The model under review builds one solid part; all positions refer to its coordinate system, in mm. A direction names the side the tool comes from. Round coordinates to 2 decimals unless told otherwise and drop trailing zeros. Order: outer loops, then holes, each group sorted by start corner. A loop starts at its lowest first (then second) coordinate and runs counter-clockwise, first axis right, second up.
```python
from build123d import *

# Parameters (mm, degrees)
BOSS_EXTRUDE1_DEPTH = 16
CUT_EXTRUDE1_REACH  = 72.897
SKETCH3_R           = 1.75
FILLET1_R           = 2


with BuildPart() as part:
    # Sketch2 → Boss-Extrude1 (new body)
    with BuildSketch(Plane.YZ):
        with BuildLine():
            Line((0, 0), (0, 20.06238879))
            ThreePointArc((0, 20.06238879), (-19, 39.06238879), (-38, 20.06238879))
            Line((-38, 20.06238879), (-38, 0))
            Line((-38, 0), (-54, 0))
            Line((-54, 0), (-54, 4))
            Line((-54, 4), (-42, 4))
            Line((-42, 4), (-42, 20.06238879))
            ThreePointArc((-42, 20.06238879), (-19, 43.06238879), (4, 20.06238879))
            Line((4, 20.06238879), (4, 4))
            Line((4, 4), (16, 4))
            Line((16, 4), (16, 0))
            Line((16, 0), (0, 0))
        make_face()
    extrude(amount=BOSS_EXTRUDE1_DEPTH)

    # Sketch3 → Cut-Extrude1 (cut, up to next)
    with BuildSketch(Plane(origin=(0, 0, 0), x_dir=(1, 0, 0), z_dir=(0, 0, -1)), mode=Mode.PRIVATE) as cut_extrude1_sk1:
        with Locations(Location((8, 49, 0), (0, 0, 270))):
            Circle(SKETCH3_R)
    cut_extrude1_tool1 = extrude(cut_extrude1_sk1.sketch, amount=-CUT_EXTRUDE1_REACH, mode=Mode.PRIVATE) & part.part
    # Sketch3 → Cut-Extrude1 (cut, up to next)
    with BuildSketch(Plane(origin=(0, 0, 0), x_dir=(1, 0, 0), z_dir=(0, 0, -1)), mode=Mode.PRIVATE) as cut_extrude1_sk2:
        with Locations(Location((8, -11, 0), (0, 0, 270))):
            Circle(SKETCH3_R)
    cut_extrude1_tool2 = extrude(cut_extrude1_sk2.sketch, amount=-CUT_EXTRUDE1_REACH, mode=Mode.PRIVATE) & part.part
    add(cut_extrude1_tool1.solids().sort_by_distance((8, -49, 0))[0], mode=Mode.SUBTRACT)
    add(cut_extrude1_tool2.solids().sort_by_distance((8, 11, 0))[0], mode=Mode.SUBTRACT)

    # Fillet1
    fillet1_edges = [part.edges().sort_by_distance(p)[0] for p in [
        (8, -42, 4),
        (8, 4, 4),
    ]]
    fillet(fillet1_edges, radius=FILLET1_R)


solid = part.part
```
(1) Consider section A-A (z = 15.5). Write out the cut boundary in (x, y).
Data:
outline: (0, -42) - (16, -42) - (16, -38) - (0, -38) - close; (0, 0) - (16, 0) - (16, 4) - (0, 4) - close
(2) Insertion check: pin 1 (4 mm diameter, centred on x = 7.5, y = -35.5, fed in from +Z); pin 2 (3 mm diameter, centred on x = 8, y = 11, fed in from -Z); pin 3 (5 mm diameter, centred on x = 6, y = -34, fed in from -Z); pin 4 (1.5 mm diameter, centred on x = 8, z = 35.5, fed in from +Y). Each pin has a flat end and moves straight along its axis. Give the tip position at first contact, or say it passes through.
Data:
pin 1: stops at z = 37.92
pin 2: passes through
pin 3: stops at z = 27.46
pin 4: stops at y = -1.3
(3) Consider section B-B (y = -49). Write out the cut boundary in (x, z), and give its area (3 significant figures).
Data:
outline: (0, 0) - (6.25, 0) - (6.25, 4) - (0, 4) - close; (9.75, 0) - (16, 0) - (16, 4) - (9.75, 4) - close
area: 50.0 mm2
(4) For faces 1 (the flat face through (6, 11, 4)), 2 (the flat face through (8, -42, 13)), 3 (the flat face through (8, -38, 10)), list the 3-axis set-ups (+Z, -Z, +X, -X, +Y, -Y) from which the entire face can be reached by the end or side of a thin tool; tool diameter is ignored.
Data:
face 1: +Z, +X, -X, +Y
face 2: +Z, +X, -X, -Y
face 3: -Z, +X, -X
(5) Consider section D-D (y = -19). Write out the cut boundary in (x, z).
Data:
outline: (0, 39.06) - (16, 39.06) - (16, 43.06) - (0, 43.06) - close
(6) Consider section C-C (x = 5.5). Write out the cut boundary in (y, z).
Data:
outline: (-54, 0) - (-38, 0) - (-38, 20.06) arc R19 cw to (0, 20.06) - (0, 0) - (16, 0) - (16, 4) - (6, 4) arc R2 cw to (4, 6) - (4, 20.06) arc R23 ccw to (-42, 20.06) - (-42, 6) arc R2 cw to (-44, 4) - (-54, 4) - close
(7) To check wall thickness, follow probe 1 along X at (y, z) = (-49, 1); probe 2 along Y at (x, z) = (15, 2); probe 3 along Y at (x, z) = (2, 10.5). State the ranges of each line that lie inside material, in increasing order.
Data:
probe 1: x = 0 to 6.25, 9.75 to 16
probe 2: y = -54 to -38, 0 to 16
probe 3: y = -42 to -38, 0 to 4
(8) Draft analysis for pull direction X (two halves, no side actions). For faces 4 (the flat face through (16, -8, 36)), 5 (the cylindrical face through (7.888, -18.582, 39.058)), 6 (the cylindrical face through (8.526, -47.331, 1.972)), state which applies: pulls with the +X half, pulls with the -X half, needs draft (parallel to the pull), parting line crosses it, or undercut.
Data:
face 4: pulls with the +X half
face 5: needs draft
face 6: undercut
